from build123d import *

# Parameters (mm, degrees)
BOSS_EXTRUDE1_START                    = 1.27
SKETCH1_W                              = 38.1
SKETCH1_H                              = 6.35
BOSS_EXTRUDE1_DEPTH                    = 20.586143
CUT_EXTRUDE1_DEPTH                     = 16.351018574
F_1_8_0_125_DIAMETER_HOLE1_D           = 3.175
F_1_8_0_125_DIAMETER_HOLE1_CSINK_D     = 4.445
F_1_8_0_125_DIAMETER_HOLE1_CSINK_ANGLE = 100
F_4_40_TAPPED_HOLE1_D                  = 2.2606
CUT_EXTRUDE2_DEPTH                     = 21.586143296


with BuildPart() as part:
    # Sketch1 → Boss-Extrude1 (new body)
    with BuildSketch(Plane.XY.offset(BOSS_EXTRUDE1_START)):
        with Locations((-57.517034371, -71.715312393)):
            Rectangle(SKETCH1_W, SKETCH1_H)
        Polygon((-62.686491947, -59.823500591), (-76.567034371, -68.540312393), (-59.530062968, -68.540312393), (-61.189226937, -59.539293818), align=None)
        Polygon((-59.530062968, -68.540312393), (-76.567034371, -68.540312393), (-76.567034371, -74.890312393), (-38.467034371, -74.890312393), (-38.467034371, -68.540312393), align=None)
    extrude(amount=BOSS_EXTRUDE1_DEPTH)

    # Sketch2 → Cut-Extrude1 (cut, through all)
    with BuildSketch(Plane(origin=(26.553910442, -74.890312393, 0), x_dir=(1, 0, 0), z_dir=(0, 1, 0))):
        with BuildLine():
            Line((-103.120944813, -13.150571648), (-93.595944813, -13.150571648))
            ThreePointArc((-93.595944813, -13.150571648), (-92.008444813, -11.563071648), (-93.595944813, -9.975571648))
            Line((-93.595944813, -9.975571648), (-103.120944813, -9.975571648))
            ThreePointArc((-103.120944813, -9.975571648), (-104.708444813, -11.563071648), (-103.120944813, -13.150571648))
        make_face()
    extrude(amount=CUT_EXTRUDE1_DEPTH, mode=Mode.SUBTRACT)

    # 1/8 (0.125) Diameter Hole1 (through all)
    with Locations(Plane.XY.offset(21.856143296)):
        with Locations((-71.901359776, -71.715312393)):
            CounterSinkHole(F_1_8_0_125_DIAMETER_HOLE1_D / 2, F_1_8_0_125_DIAMETER_HOLE1_CSINK_D / 2, counter_sink_angle=F_1_8_0_125_DIAMETER_HOLE1_CSINK_ANGLE)

    # #4-40 Tapped Hole1 (through all)
    with Locations(Plane.XY.offset(21.856143296)):
        with Locations((-41.921434371, -71.715312393)):
            Hole(F_4_40_TAPPED_HOLE1_D / 2)

    # Sketch7 → Cut-Extrude2 (cut, through all)
    with BuildSketch(Plane.XY.offset(21.856143296)):
        with BuildLine():
            Line((-53.867665963, -71.139758797), (-56.407665963, -71.139758797))
            ThreePointArc((-56.407665963, -71.139758797), (-59.582665963, -67.964758797), (-56.407665963, -64.789758797))
            Line((-56.407665963, -64.789758797), (-53.867665963, -64.789758797))
            ThreePointArc((-53.867665963, -64.789758797), (-50.692665963, -67.964758797), (-53.867665963, -71.139758797))
        make_face()
    extrude(amount=-CUT_EXTRUDE2_DEPTH, mode=Mode.SUBTRACT)


solid = part.part
Read the model definition and answer for the solid it produces. Units are mm, in the model's axes. A direction names the side the tool comes from. Coordinates: 2 decimals unless noted, no trailing zeros. Loops run counter-clockwise (first coordinate to the right, second up) from the corner with the lowest first, then second, coordinate; pieces in that order, holes last. Notation, with made-up numbers: (65.5, 15.25) -> (77.5, 15.25) arc R29 cw to (77.5, 39.25) -> close; hole circle Ø7 at (64.25, 68.25). An arc over 180 degrees is marked (long way). Answer in a Markdown table with one row per item.
Item 1: Each of these flat-tipped pins is pushed along its axis until it touches: P1, Ø10, axis at x = -45.5, z = 15, coming from the +Y side; P2, Ø1.5, axis at y = -65, z = 17, coming from the -X side; P3, Ø1.9, axis at x = -71.9, y = -71.72, coming from the -Z side; P4, Ø2, axis at x = -55, z = 11, coming from the +Y side. Where does it stop, or does it pass through?
Returned:
| item | result |
|---|---|
| P1 | stops at y = -68.54 |
| P2 | stops at x = -72.12 |
| P3 | passes through |
| P4 | stops at y = -71.14 |
Item 2: For a pull along Z with two mould halves and no side action, classify faces 6 (the flat face through (-69.5, -64.1, 9.1)), 7 (the flat face through (-58, -72, 21.856)), 8 (the flat face through (-62, -71, 1.27)), 9 (the flat face through (-71, -70, 9.976)) as released by +Z, released by -Z, zero draft, split by the parting line, or undercut.
Returned:
| item | result |
|---|---|
| face 6 | zero draft |
| face 7 | released by +Z |
| face 8 | released by -Z |
| face 9 | undercut |
Item 3: A cutting plane is placed at D-D on z = 4. Give the number of separate pieces and of enclosed holes in the cut face, plus the area to 3 significant figures.
Returned:
| item | result |
|---|---|
| separate pieces | 1 |
| enclosed holes | 2 |
| area | 292 mm^2 |
Item 4: A cutting plane is placed at C-C on y = -65.25. Determine the outline of the cut face in (x, z) (1 decimal), plus the area to 3 significant figures.
Returned:
| item | result |
|---|---|
| outline | (-71.3, 1.3) -> (-60.1, 1.3) -> (-60.1, 21.9) -> (-71.3, 21.9) -> (-71.3, 13.2) -> (-67, 13.2) arc R1.6 cw to (-67, 10) -> (-71.3, 10) -> close |
| area | 213 mm^2 |
Item 5: For faces 1 (the flat face through (-71, -70, 13.151)), 2 (the flat face through (-38.467, -72, 11)), 3 (the flat face through (-76.567, -72, 6)), 4 (the flat face through (-45, -68.54, 11)), 5 (the cylindrical face through (-51.813, -70.385, 11.707)), determine the directions among +Z, -Z, +X, -X, +Y, -Y from which every point of the face is accessible in a straight line to the end or side of a thin tool.
Returned:
| item | result |
|---|---|
| face 1 | -X, +Y, -Y |
| face 2 | +Z, -Z, +X, +Y, -Y |
| face 3 | +Z, -Z, -X, +Y, -Y |
| face 4 | +Z, -Z, +X, +Y |
| face 5 | +Z, -Z, +Y |
Item 6: Straight lines are drawn through the part: line 1 along X through (y, z) = (-71.75, 15.5); line 2 along X through (y, z) = (-71.25, 9); line 3 along Y through (x, z) = (-46, 19.5). For each, find the intervals that lie inside material, in ascending order. Write a range as [from, to].
Returned:
| item | result |
|---|---|
| line 1 | x = [-76.57, -73.49], [-70.31, -43.05], [-40.79, -38.47] |
| line 2 | x = [-76.57, -73.42], [-70.38, -42.95], [-40.89, -38.47] |
| line 3 | y = [-74.89, -68.54] |
Item 7: A cutting plane is placed at B-B on x = -67.5. Determine the outline of the cut face in (y, z), plus the area to 3 significant figures.
Returned:
| item | result |
|---|---|
| outline | (-74.89, 1.27) -> (-62.85, 1.27) -> (-62.85, 9.98) -> (-74.89, 9.98) -> close; (-74.89, 13.15) -> (-62.85, 13.15) -> (-62.85, 21.86) -> (-74.89, 21.86) -> close |
| area | 210 mm^2 |
